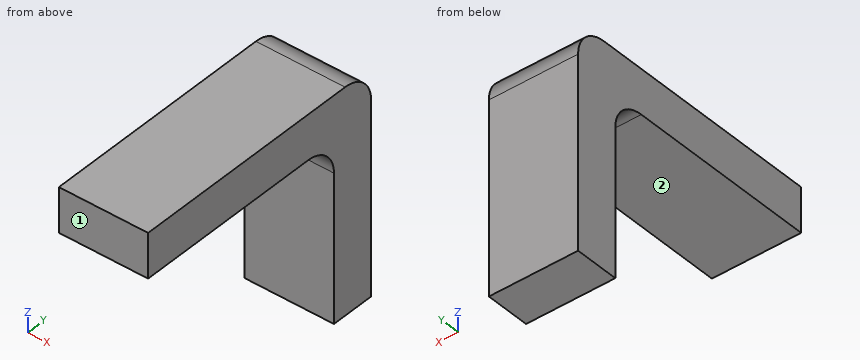
from build123d import *

# Parameters (mm, degrees)
F0_W     = 20
F0_H     = 50
F1_DEPTH = 10
F2_W     = 20
F2_H     = 10
F3_DEPTH = 50
F4_R     = 7


with BuildPart() as f1:
    # F0 (on Front) → F1 (new body)
    with BuildSketch(Plane.XZ):
        with Locations((10, 25)):
            Rectangle(F0_W, F0_H)
    extrude(amount=F1_DEPTH)

    # F2 (on face) → F3 (join)
    with BuildSketch(Plane.XZ.offset(10)):
        with Locations((10, 45)):
            Rectangle(F2_W, F2_H)
    extrude(amount=F3_DEPTH)

    # F4
    f4_edges = [f1.edges().sort_by_distance(p)[0] for p in [
        (10, 0, 50),
        (10, -10, 40),
    ]]
    fillet(f4_edges, radius=F4_R)


solid = f1.part
For this review, take the finished solid that the model builds, in its own axes (mm). Face numbers are marked on the shaded views. A direction names the side the tool comes from. Coordinates: 2 decimals unless noted, no trailing zeros. Order: outer loops, then holes, each group sorted by start corner. A loop starts at its lowest first (then second) coordinate and runs counter-clockwise, first axis right, second up. Notation, with made-up numbers: (-40, 66.5) - (-21, 66.5) arc R5 cw to (-21, 74.5) - close; hole circle Ø5 at (57.25, -12). An arc over 180 degrees is marked (long way). Answer as CSV lines item,"result". Start each with the question number.
1) Add section B-B (z = 26). State the section outline as (x, y) points, then the cut area to 3 significant figures.
2) To check wall thickness, follow line 1 along Y through (x, z) = (6.25, 13); line 2 along Z through (x, y) = (7, -23.5); line 3 along Z through (x, y) = (5.5, -14.5). State the ranges of each line that lie inside material, in increasing order. Write a range as [from, to].
3) Add section C-C (y = -50). State the section outline as (x, z) points.
4) Add section A-A (x = 1.5). State the section outline as (y, z) points, then the cut area to 3 significant figures.
5) Machinability: for the marked faces 1 and 2, which of the approach directions +Z, -Z, +X, -X, +Y, -Y give a long, thin tool a straight path to every point of the face, cutting with its end or side? Answer none if there is none.
6) Insertion check: P1, Ø10, axis at x = 9.5, y = -34, coming from the -Z side. The pin has a flat end and moves straight along its axis. Give the tip position at first contact, or say it passes through.
Result:
1,outline,"(0, -10) - (20, -10) - (20, 0) - (0, 0) - close"
1,area,"200 mm^2"
2,line 1,"[-10, 0]"
2,line 2,"[40, 50]"
2,line 3,"[39.54, 50]"
3,outline,"(0, 40) - (20, 40) - (20, 50) - (0, 50) - close"
4,outline,"(-60, 40) - (-17, 40) arc R7 cw to (-10, 33) - (-10, 0) - (0, 0) - (0, 43) arc R7 ccw to (-7, 50) - (-60, 50) - close"
4,area,"1,000 mm^2"
5,face 1,"+Z, -Z, +X, -X, -Y"
5,face 2,"-Z, +X, -X, -Y"
6,P1,"z = 40"
